Design review of the part built by this model. Coordinates are the model's own, in mm. Face numbers are marked on the shaded views. Give positions to 0.01 mm unless a question says otherwise; leave off trailing zeros. Loops run counter-clockwise (first coordinate to the right, second up) from the corner with the lowest first, then second, coordinate; pieces in that order, holes last. Notation, with made-up numbers: (89.5, 24.25) - (141.5, 24.25) arc R35 ccw to (141.5, 57.25) - close; hole circle Ø8 at (-2.75, 11.5). An arc over 180 degrees is marked (long way). Write each question's results on one line, items separated by ' | '.
```python
from build123d import *

# Parameters (mm, degrees)
BOSS_EXTRUDE1_DEPTH = 10
SKETCH2_R           = 7.6
BOSS_EXTRUDE2_DEPTH = 10
SKETCH4_R           = 12
CUT_EXTRUDE2_DEPTH  = 77.40353395


with BuildPart() as part:
    # Sketch1 → Boss-Extrude1 (new body)
    with BuildSketch(Plane(origin=(0, 0, 0), x_dir=(0, 1, 0), z_dir=(0, 0, 1))):
        with BuildLine():
            Line((-25, -37.5), (25, -37.5))
            ThreePointArc((25, -37.5), (33.838834765, -33.838834765), (37.5, -25))
            Line((37.5, -25), (37.5, 25))
            ThreePointArc((37.5, 25), (33.838834765, 33.838834765), (25, 37.5))
            Line((25, 37.5), (-25, 37.5))
            ThreePointArc((-25, 37.5), (-33.838834765, 33.838834765), (-37.5, 25))
            Line((-37.5, 25), (-37.5, -25))
            ThreePointArc((-37.5, -25), (-33.838834765, -33.838834765), (-25, -37.5))
        make_face()
    extrude(amount=BOSS_EXTRUDE1_DEPTH)

    # Sketch2 → Boss-Extrude2 (add)
    with BuildSketch(Plane.YZ.offset(37.5)):
        with BuildLine():
            ThreePointArc((14.587782351, 53.492363969), (0, 65), (-14.587782351, 53.492363969))
            Line((-14.587782351, 53.492363969), (-25, 10))
            Line((-25, 10), (25, 10))
            Line((25, 10), (14.587782351, 53.492363969))
        make_face()
        with Locations(Location((0, 50, 0), (0, 0, 270))):
            Circle(SKETCH2_R, mode=Mode.SUBTRACT)
    boss_extrude2 = extrude(amount=-BOSS_EXTRUDE2_DEPTH)

    # Mirror1: Boss-Extrude2 across plane
    add(boss_extrude2.mirror(Plane(origin=(0, 0, 0), x_dir=(0, 0, 1), z_dir=(1, 0, 0))))

    # Sketch4 → Cut-Extrude2 (cut, through all)
    with BuildSketch(Plane.XY.offset(10)):
        Circle(SKETCH4_R)
    extrude(amount=-CUT_EXTRUDE2_DEPTH, mode=Mode.SUBTRACT)


solid = part.part
```
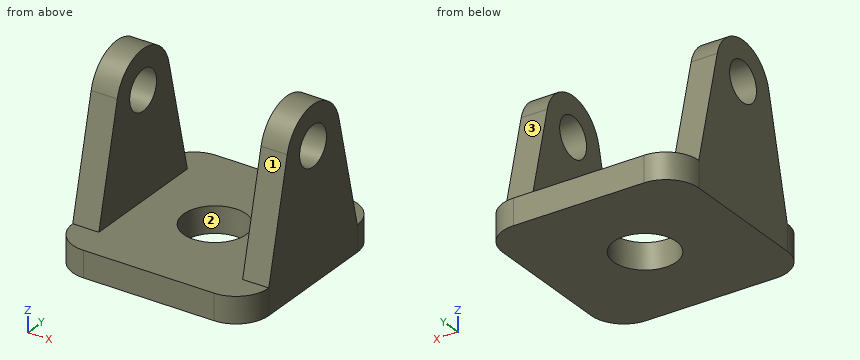
Item 1: Wall thickness on probe 1 along X at (y, z) = (-1, 62); probe 2 along Y at (x, z) = (0, 2.5); probe 3 along Z at (x, y) = (-22.5, 29.5): over which ranges is each line inside the solid? List them lowest first.
Output values:
probe 1: x = -37.5 to -27.5, 27.5 to 37.5 | probe 2: y = -37.5 to -12, 12 to 37.5 | probe 3: z = 0 to 10
Item 2: Clearance check with flat-ended pins moving along their axes: P1, Ø12, axis at x = -29, z = 49.5, coming from the +Y side; P2, Ø10, axis at x = -27, z = 27.5, coming from the +Y side; P3, Ø5, axis at x = -17, y = 26, coming from the +Z side. State where each tip first meets the part, or that it passes through.
Output values:
P1: stops at y = 16.98 | P2: stops at y = 22 | P3: stops at z = 10
Item 3: We need section D-D on z = 17. Give the boundary of the cut face in (x, y), then the cut area to 3 significant figures.
Output values:
outline: (-37.5, -23.32) - (-27.5, -23.32) - (-27.5, 23.32) - (-37.5, 23.32) - close; (27.5, -23.32) - (37.5, -23.32) - (37.5, 23.32) - (27.5, 23.32) - close | area: 933 mm²
Item 4: We need section B-B on y = 0. Give the boundary of the cut face in (x, z).
Output values:
outline: (-37.5, 0) - (-12, 0) - (-12, 10) - (-27.5, 10) - (-27.5, 42.4) - (-37.5, 42.4) - close; (-37.5, 57.6) - (-27.5, 57.6) - (-27.5, 65) - (-37.5, 65) - close; (12, 0) - (37.5, 0) - (37.5, 42.4) - (27.5, 42.4) - (27.5, 10) - (12, 10) - close; (27.5, 57.6) - (37.5, 57.6) - (37.5, 65) - (27.5, 65) - close
Item 5: We need section A-A on z = 50. Give the boundary of the cut face in (x, y).
Output values:
outline: (-37.5, -15.42) - (-27.5, -15.42) - (-27.5, -7.6) - (-37.5, -7.6) - close; (-37.5, 7.6) - (-27.5, 7.6) - (-27.5, 15.42) - (-37.5, 15.42) - close; (27.5, -15.42) - (37.5, -15.42) - (37.5, -7.6) - (27.5, -7.6) - close; (27.5, 7.6) - (37.5, 7.6) - (37.5, 15.42) - (27.5, 15.42) - close
Item 6: Draft analysis for pull direction Y (two halves, no side actions). For the marked faces 1, 2 and 3, state which applies: +Y half, -Y half, draft (parallel to the pull), parting line (faces both ways), or undercut.
Output values:
face 1: -Y half | face 2: undercut | face 3: +Y half
Item 7: We need section C-C on x = 0. Give the boundary of the cut face in (y, z).
Output values:
outline: (-37.5, 0) - (-12, 0) - (-12, 10) - (-37.5, 10) - close; (12, 0) - (37.5, 0) - (37.5, 10) - (12, 10) - close
